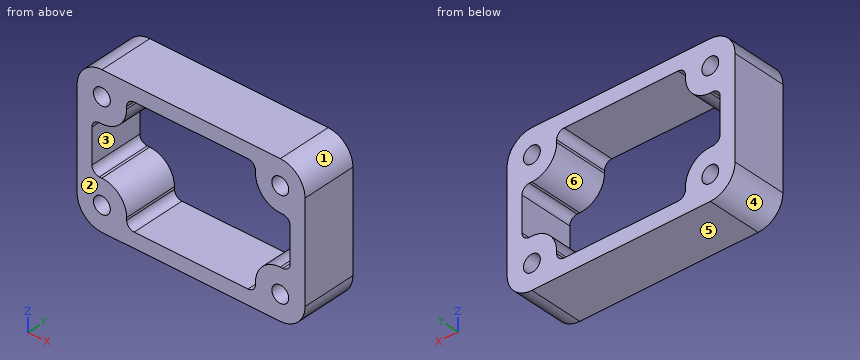
```python
from build123d import *

# Parameters (mm, degrees)
SKETCH006_W = 46
SKETCH006_H = 30
SKETCH006_R = 1.7
PAD_DEPTH   = 11
FILLET_R    = 5
FILLET001_R = 5
FILLET002_R = 5
FILLET003_R = 5
FILLET004_R = 5
FILLET005_R = 5
FILLET006_R = 5
FILLET007_R = 5
FILLET008_R = 1.5
FILLET009_R = 1.5
FILLET010_R = 1.5
FILLET011_R = 1.5
FILLET012_R = 1.5
FILLET013_R = 1.5
FILLET014_R = 1.5
FILLET015_R = 1.5


with BuildPart() as part:
    # Sketch006 → Pad (new body)
    with BuildSketch(Plane(origin=(0, 25, 0), x_dir=(-1, 0, 0), z_dir=(0, 1, 0))):
        with Locations((0, 30)):
            Rectangle(SKETCH006_W, SKETCH006_H)
        with Locations((-18, 20)):
            Circle(SKETCH006_R, mode=Mode.SUBTRACT)
        with Locations((18, 20)):
            Circle(SKETCH006_R, mode=Mode.SUBTRACT)
        with Locations((-18, 40)):
            Circle(SKETCH006_R, mode=Mode.SUBTRACT)
        with Locations((18, 40)):
            Circle(SKETCH006_R, mode=Mode.SUBTRACT)
        Polygon((-13, 35), (-13, 42), (13, 42), (13, 35), (20, 35), (20, 25), (13, 25), (13, 18), (-13, 18), (-13, 25), (-20, 25), (-20, 35), align=None, mode=Mode.SUBTRACT)
    extrude(amount=PAD_DEPTH)

    # Fillet
    fillet_edges = [part.edges().sort_by_distance(p)[0] for p in [
        (23, 30.5, 45),
    ]]
    fillet(fillet_edges, radius=FILLET_R)

    # Fillet001
    fillet001_edges = [part.edges().sort_by_distance(p)[0] for p in [
        (23, 30.5, 15),
    ]]
    fillet(fillet001_edges, radius=FILLET001_R)

    # Fillet002
    fillet002_edges = [part.edges().sort_by_distance(p)[0] for p in [
        (-23, 30.5, 15),
    ]]
    fillet(fillet002_edges, radius=FILLET002_R)

    # Fillet003
    fillet003_edges = [part.edges().sort_by_distance(p)[0] for p in [
        (-23, 30.5, 45),
    ]]
    fillet(fillet003_edges, radius=FILLET003_R)

    # Fillet004
    fillet004_edges = [part.edges().sort_by_distance(p)[0] for p in [
        (13, 30.5, 25),
    ]]
    fillet(fillet004_edges, radius=FILLET004_R)

    # Fillet005
    fillet005_edges = [part.edges().sort_by_distance(p)[0] for p in [
        (13, 30.5, 35),
    ]]
    fillet(fillet005_edges, radius=FILLET005_R)

    # Fillet006
    fillet006_edges = [part.edges().sort_by_distance(p)[0] for p in [
        (-13, 30.5, 35),
    ]]
    fillet(fillet006_edges, radius=FILLET006_R)

    # Fillet007
    fillet007_edges = [part.edges().sort_by_distance(p)[0] for p in [
        (-13, 30.5, 25),
    ]]
    fillet(fillet007_edges, radius=FILLET007_R)

    # Fillet008
    fillet008_edges = [part.edges().sort_by_distance(p)[0] for p in [
        (-13, 30.5, 42),
    ]]
    fillet(fillet008_edges, radius=FILLET008_R)

    # Fillet009
    fillet009_edges = [part.edges().sort_by_distance(p)[0] for p in [
        (13, 30.5, 42),
    ]]
    fillet(fillet009_edges, radius=FILLET009_R)

    # Fillet010
    fillet010_edges = [part.edges().sort_by_distance(p)[0] for p in [
        (20, 30.5, 35),
    ]]
    fillet(fillet010_edges, radius=FILLET010_R)

    # Fillet011
    fillet011_edges = [part.edges().sort_by_distance(p)[0] for p in [
        (20, 30.5, 25),
    ]]
    fillet(fillet011_edges, radius=FILLET011_R)

    # Fillet012
    fillet012_edges = [part.edges().sort_by_distance(p)[0] for p in [
        (13, 30.5, 18),
    ]]
    fillet(fillet012_edges, radius=FILLET012_R)

    # Fillet013
    fillet013_edges = [part.edges().sort_by_distance(p)[0] for p in [
        (-20, 30.5, 35),
    ]]
    fillet(fillet013_edges, radius=FILLET013_R)

    # Fillet014
    fillet014_edges = [part.edges().sort_by_distance(p)[0] for p in [
        (-13, 30.5, 18),
    ]]
    fillet(fillet014_edges, radius=FILLET014_R)

    # Fillet015
    fillet015_edges = [part.edges().sort_by_distance(p)[0] for p in [
        (-20, 30.5, 25),
    ]]
    fillet(fillet015_edges, radius=FILLET015_R)


solid = part.part
```
CAD build for the part. Positions are in the model's coordinates, mm. Face numbers are marked on the shaded views. A direction names the side the tool comes from. Round coordinates to 2 decimals unless told otherwise and drop trailing zeros. Order: outer loops, then holes, each group sorted by start corner. A loop starts at its lowest first (then second) coordinate and runs counter-clockwise, first axis right, second up. Notation, with made-up numbers: (18.25, -16.75) - (26.25, -16.75) arc R15 cw to (26.25, 0.25) - close; hole circle Ø4 at (23.25, -20.5). An arc over 180 degrees is marked (long way). Answer in a Markdown table with one row per item. Add a question column.
(1) Band-saw the part on B-B on z = 23. List the corners of the cut face in (x, y).
(2) Band-saw the part on A-A on x = 9.5. List the corners of the cut face in (y, z).
(3) Probe L1, parallel to Z at x = -18, y = 31; L2, parallel to X at y = 30, z = 27.5; L3, parallel to X at y = 32.5, z = 19.75. List the from-to ranges inside material, lowest first. Write a range as [from, to].
(4) Drop a flat-ended pin along its axis: pin 1 Ø0.6 at (x, y) = (18.5, 32.5) entering from +Z. Give the stop position or say it passes through.
(5) Band-saw the part on C-C on y = 28.5. Count the separate pieces of the cut face and the enclosed holes in it, and give its area (3 significant figures).
(6) Mould opens along Z. For the marked faces 1, 2, 3 and 4 say: +Z half, -Z half, draft (parallel to the pull), parting line (faces both ways), or undercut.
(7) 3-axis set-ups, long thin cutter, end or side, ignore diameter. For the marked faces 5 and 6: which of +Z, -Z, +X, -X, +Y, -Y reach the whole face in a straight line?
Data:
| question | item | result |
|---|---|---|
| 1 | outline | (-23, 25) - (-14, 25) - (-14, 36) - (-23, 36) - close; (14, 25) - (23, 25) - (23, 36) - (14, 36) - close |
| 2 | outline | (25, 15) - (36, 15) - (36, 18) - (25, 18) - close; (25, 42) - (36, 42) - (36, 45) - (25, 45) - close |
| 3 | L1 | z = [15, 18.3], [21.7, 25], [35, 38.3], [41.7, 45] |
| 3 | L2 | x = [-23, -20], [20, 23] |
| 3 | L3 | x = [-22.99, -19.68], [-16.32, -13], [13, 16.32], [19.68, 22.99] |
| 4 | pin 1 | stops at z = 45 |
| 5 | separate pieces | 1 |
| 5 | enclosed holes | 5 |
| 5 | area | 541 mm^2 |
| 6 | face 1 | +Z half |
| 6 | face 2 | draft |
| 6 | face 3 | undercut |
| 6 | face 4 | -Z half |
| 7 | face 5 | -Z, +X, -X, +Y, -Y |
| 7 | face 6 | +Y, -Y |
